Build history of the part. All positions in model axes, mm. Coordinates: 2 decimals unless noted, no trailing zeros. Order: outer loops, then holes, each group sorted by start corner. A loop starts at its lowest first (then second) coordinate and runs counter-clockwise, first axis right, second up. Notation, with made-up numbers: (42.5, 64.5) -> (54.5, 64.5) arc R9 cw to (54.5, 70.5) -> close; hole circle Ø2 at (82.5, 89.25). An arc over 180 degrees is marked (long way). Write each question's results on one line, items separated by ' | '.
Autodesk Fusion 360 part; units mm, degrees
sketch "Sketch1" plane through (0, 0, 0) normal (0, 0, 1) x (1, 0, 0)
  circle A0 centre (0, 0) radius 37.5
  circle A1 centre (0, 0) radius 32.5
  circle A2 centre (0, 0) radius 36.5
  line L0 (-18, 0) -> (18, 0)
  line L1 (18, 0) -> (18, -31.753)
  line L2 (-18, 0) -> (-18, -31.753)
  line L3 (45, -45) -> (-45, -45)
  line L4 (-45, -45) -> (-45, 45)
  line L5 (-45, 45) -> (45, 45)
  line L6 (45, 45) -> (45, -45)
  line L7 (45, -45) -> (-45, 45) construction
  line L8 (-45, -45) -> (45, 45) construction
  dimension "d1" = 75
  dimension "d2" = -5
  dimension "d3" = -1
  dimension "d4" = 36
  dimension "d5" = 90
  dimension "d6" = 90
extrude "Extrude1" add sketch "Sketch1" along normal blind 5 contours L3 L4 L5 L6
extrude "Extrude2" add sketch "Sketch1" along normal blind 3 contours A0 | A1 A2 L1 L2 picked at (-19.5132, -29.1741)
chamfer "Chamfer1" distance 14 angle 45 4 edges at (-45, 45, 2.5) (45, 45, 2.5) (45, -45, 2.5) (-45, -45, 2.5)
fillet "Fillet1" radius 10 8 edges at (-31, 45, 2.5) (-45, 31, 2.5) (31, 45, 2.5) (45, 31, 2.5) (45, -31, 2.5) (31, -45, 2.5) (-31, -45, 2.5) (-45, -31, 2.5)
sketch "Sketch2" plane through (0, 0, 0) normal (0, 0, 1) x (1, 0, 0)
  line L0 (33, -33) -> (-33, -33)
  line L1 (-33, -33) -> (-33, 33)
  line L2 (-33, 33) -> (33, 33)
  line L3 (33, 33) -> (33, -33)
  line L4 (33, -33) -> (-33, 33) construction
  line L5 (-33, -33) -> (33, 33) construction
  dimension "d14" = 66
  dimension "d15" = 66
hole "Hole1" at (33, 33, 0) at (33, -33, 0) at (-33, -33, 0) at (-33, 33, 0) direction (0, 0, 1) diameter 2.5 depth 5 tip angle 180
chamfer "Chamfer2" distance 0.8 angle 45 16 edges at (0, 45, 5) (-30.6847, 44.2388, 5) (-38, 38, 5) (-44.2388, 30.6847, 5) (-45, 0, 5) (-44.2388, -30.6847, 5) (-38, -38, 5) (-30.6847, -44.2388, 5) (0, -45, 5) (30.6847, -44.2388, 5) (38, -38, 5) (44.2388, -30.6847, 5) (45, 0, 5) (44.2388, 30.6847, 5) (38, 38, 5) (30.6847, 44.2388, 5)
chamfer "Chamfer2" distance 0.8 angle 45 1 edges at (-34.9623, 13.5606, 5)
chamfer "Chamfer2" distance 1 angle 45 4 edges at (34.1654, 32.548, 5) (34.1654, -33.452, 5) (-31.8346, -33.452, 5) (-31.8346, 32.548, 5)
fillet "Fillet2" radius 2 4 edges at (-18, -31.753, 1.5) (-18, -27.0601, 1.5) (18, -31.753, 1.5) (18, -27.0601, 1.5)
Item 1: Drill centre lines: line 1 (X direction, y = -33, z = 1.8); line 2 (Y direction, x = 33, z = 1.9); line 3 (Y direction, x = 33, z = 3.1). Where is each one in solid material? Low to high. Write a range as from..to.
Answer:
line 1: x = -42.89..-34.25, -31.75..-15.6, 15.6..31.75, 34.25..42.89 | line 2: y = -42.89..-34.25, -31.75..31.75, 34.25..42.89 | line 3: y = -42.89..-34.25, -31.75..-17.81, 17.81..31.75, 34.25..42.89
Item 2: Pull direction X, two halves, no side cores. Call faces 1 (the conical face through (-43.772, -30.548, 4.683)), 2 (the cylindrical face through (-32.521, -31.845, 2.028)), 3 (the flat face through (0, -45, 2)): released by +X, released by -X, zero draft, split by the parting line, or undercut.
Answer:
face 1: released by -X | face 2: undercut | face 3: zero draft
Item 3: Slice it at B-B, the plane y = 0. List the corners of the cut face in (x, z), and give its area (3 significant figures).
Answer:
outline: (-45, 0) -> (-32.5, 0) -> (-32.5, 3) -> (-37.5, 3) -> (-37.5, 4.2) -> (-38.3, 5) -> (-44.2, 5) -> (-45, 4.2) -> close; (32.5, 0) -> (45, 0) -> (45, 4.2) -> (44.2, 5) -> (38.3, 5) -> (37.5, 4.2) -> (37.5, 3) -> (32.5, 3) -> close | area: 104 mm^2
Item 4: Pin check, flat tips, straight feed: pin 1 (8 mm diameter, centred on x = 17.5, y = 24.5, fed in from +Z); pin 2 (2.5 mm diameter, centred on y = -29.5, z = 1.5, fed in from +X); pin 3 (0.7 mm diameter, centred on y = -29, z = 2, fed in from -X). Stop position of each tip, or through.
Answer:
pin 1: stops at z = 3 | pin 2: stops at x = 44.9 | pin 3: stops at x = -44.84
Item 5: Slice it at A-A, the plane z = 2.05. List the corners of the cut face in (x, y), and give its area (3 significant figures).
Answer:
outline: (-45, -26.86) arc R10 ccw to (-42.07, -33.93) -> (-33.93, -42.07) arc R10 ccw to (-26.86, -45) -> (26.86, -45) arc R10 ccw to (33.93, -42.07) -> (42.07, -33.93) arc R10 ccw to (45, -26.86) -> (45, 26.86) arc R10 ccw to (42.07, 33.93) -> (33.93, 42.07) arc R10 ccw to (26.86, 45) -> (-26.86, 45) arc R10 ccw to (-33.93, 42.07) -> (-42.07, 33.93) arc R10 ccw to (-45, 26.86) -> close; hole circle Ø2.5 at (-33, -33); hole circle Ø2.5 at (-33, 33); hole (-18.84, -26.48) arc R2 cw to (-18, -28.11) -> (-18, -30.57) arc R2 ccw to (-16.93, -32.34) arc R36.5 ccw to (16.93, -32.34) arc R2 ccw to (18, -30.57) -> (18, -28.11) arc R2 cw to (18.84, -26.48) arc R32.5 ccw (long way) to start; hole circle Ø2.5 at (33, -33); hole circle Ø2.5 at (33, 33) | area: 4,200 mm^2
